Check sheet for the modelled part. Datum: model origin and axes. Units: mm. A direction names the side the tool comes from. Give positions to 0.01 mm unless a question says otherwise; leave off trailing zeros. Write each loop counter-clockwise with the first axis right and the second up, starting at its lowest first coordinate (ties: lowest second). Pieces come first, ordered by that corner, then holes. Notation, with made-up numbers: (11.5, 7.25) -> (18.5, 7.25) arc R21 ccw to (18.5, 15.25) -> close; hole circle Ø3 at (-5.75, 2). An arc over 180 degrees is marked (long way). Use a Markdown table: item, result. Add a question column.
1. Cross-section at D-D (x = 31.5). Enter the section's corners in (y, z), then the cut area to 3 significant figures.
2. Gauge pin test, flat ends, axial feed: P1, Ø8, axis at x = -16, y = 2.5, coming from the -Z side; P2, Ø12, axis at x = -20, y = 2.5, coming from the +Z side; P3, Ø12.5, axis at x = 0, y = 0, coming from the +Z side; P4, Ø1.5, axis at y = 1.5, z = 10, coming from the -X side. Record the tip position at first contact, or that the pin passes through.
3. Release check for a two-part mould opening along Y. For faces 3 (the flat face through (-16.6, -9.3, 2.3)), 4 (the flat face through (1, 8, 4.762)), 5 (the flat face through (-19, 0, 4.762)) record: released by +Y, released by -Y, zero draft, split by the parting line, or undercut.
4. Cross-section at B-B (z = 3.5). Enter the section's corners in (x, y), then the cut area to 3 significant figures.
5. Set-up check for faces 1 (the cylindrical face through (-8.88, -2.8, 2.35)), 2 (the flat face through (-8.4, -5.4, 0)): record each of +Z, -Z, +X, -X, +Y, -Y from which the full face is reachable in a straight line by a thin tool's end or side.
6. Cross-section at A-A (x = 0). Enter the section's corners in (y, z).
7. Cross-section at C-C (y = 0). Count the separate pieces of the cut face and the enclosed holes in it, then the cut area to 3 significant figures.
8. Scan lines: probe 1 along X at (y, z) = (0.75, 2); probe 2 along Z at (x, y) = (-19, 1); probe 3 along X at (y, z) = (1, 10.5). Record each from-to range of solid material in increasing order. Write a range as [from, to].
from build123d import *

# Parameters (mm, degrees)
SKETCH1_R           = 6.604
SKETCH1_R_2         = 3.429
SKETCH1_R_3         = 12.4841
SKETCH1_R_4         = 9.3091
BOSS_EXTRUDE1_DEPTH = 4.7625
SKETCH3_R           = 12.4841
SKETCH2_R           = 9.3091
SKETCH5_R           = 7.7216
CUT_EXTRUDE1_DEPTH  = 40.575251945


with BuildPart() as part:
    # Sketch1 → Boss-Extrude1 (new body)
    # profile 1 of 5: a face of its own
    with BuildSketch(Plane.XY):
        with Locations((-28.894599, 0)):
            Circle(SKETCH1_R)
        with Locations(Location((-28.894599, 0, 0), (0, 0, 180))):
            Circle(SKETCH1_R_2, mode=Mode.SUBTRACT)
    # profile 2 of 5: a face of its own
    with BuildSketch(Plane.XY):
        with BuildLine():
            Line((-2.540535565, 12.222865124), (-30.238524223, 6.465808611))
            ThreePointArc((-30.238524223, 6.465808611), (-24.727013738, 5.1228946), (-22.290599, 0))
            ThreePointArc((-22.290599, 0), (-24.727013738, -5.1228946), (-30.238524223, -6.465808611))
            Line((-30.238524223, -6.465808611), (-2.540535565, -12.222865124))
            ThreePointArc((-2.540535565, -12.222865124), (-12.4841, 0), (-2.540535565, 12.222865124))
        make_face()
    # profile 3 of 5: a face of its own
    with BuildSketch(Plane.XY):
        Circle(SKETCH1_R_3)
        with Locations(Location((0, 0, 0), (0, 0, 180))):
            Circle(SKETCH1_R_4, mode=Mode.SUBTRACT)
    # profile 4 of 5: a face of its own
    with BuildSketch(Plane.XY):
        with BuildLine():
            Line((30.238524223, 6.465808611), (2.540535565, 12.222865124))
            ThreePointArc((2.540535565, 12.222865124), (9.684241139, 7.878339062), (12.4841, 0))
            ThreePointArc((12.4841, 0), (9.684241139, -7.878339062), (2.540535565, -12.222865124))
            Line((2.540535565, -12.222865124), (30.238524223, -6.465808611))
            ThreePointArc((30.238524223, -6.465808611), (22.290599, 0), (30.238524223, 6.465808611))
        make_face()
    # profile 5 of 5: a face of its own
    with BuildSketch(Plane.XY):
        with Locations((28.894599, 0)):
            Circle(SKETCH1_R)
        with Locations(Location((28.894599, 0, 0), (0, 0, 180))):
            Circle(SKETCH1_R_2, mode=Mode.SUBTRACT)
    extrude(amount=BOSS_EXTRUDE1_DEPTH)

    # Sketch3 → Loft3 section 0
    with BuildSketch(Plane.XY.offset(4.7625)):
        Circle(SKETCH3_R)
    # Sketch2 → Loft3 section 1
    with BuildSketch(Plane.XY.offset(12.2555)):
        Circle(SKETCH2_R)
    loft()

    # Sketch5 → Cut-Extrude1 (cut, through all)
    with BuildSketch(Plane.XY.offset(12.2555)):
        Circle(SKETCH5_R)
    extrude(amount=-CUT_EXTRUDE1_DEPTH, mode=Mode.SUBTRACT)


solid = part.part
Worked answers:
| question | item | result |
|---|---|---|
| 1 | outline | (-6.07, 0) -> (-2.23, 0) -> (-2.23, 4.76) -> (-6.07, 4.76) -> close; (2.23, 0) -> (6.07, 0) -> (6.07, 4.76) -> (2.23, 4.76) -> close |
| 1 | area | 36.6 mm² |
| 2 | P1 | stops at z = 0 |
| 2 | P2 | stops at z = 4.76 |
| 2 | P3 | passes through |
| 2 | P4 | stops at x = -10.49 |
| 3 | face 3 | released by -Y |
| 3 | face 4 | undercut |
| 3 | face 5 | zero draft |
| 4 | outline | (-30.24, -6.47) -> (-2.54, -12.22) arc R12.48 ccw to (2.54, -12.22) -> (30.24, -6.47) arc R6.6 ccw to (30.24, 6.47) -> (2.54, 12.22) arc R12.48 ccw to (-2.54, 12.22) -> (-30.24, 6.47) arc R6.6 ccw to start; hole circle Ø6.86 at (-28.89, 0); hole circle Ø18.62 at (0, 0); hole circle Ø6.86 at (28.89, 0) |
| 4 | area | 917 mm² |
| 5 | face 1 | -Z |
| 5 | face 2 | -Z, +X, -X, +Y, -Y |
| 6 | outline | (-12.48, 0) -> (-9.31, 0) -> (-9.31, 4.76) -> (-7.72, 4.76) -> (-7.72, 12.26) -> (-9.31, 12.26) -> (-12.48, 4.76) -> close; (7.72, 4.76) -> (9.31, 4.76) -> (9.31, 0) -> (12.48, 0) -> (12.48, 4.76) -> (9.31, 12.26) -> (7.72, 12.26) -> close |
| 7 | separate pieces | 4 |
| 7 | enclosed holes | 0 |
| 7 | area | 232 mm² |
| 8 | probe 1 | x = [-35.46, -32.24], [-25.55, -9.28], [9.28, 25.55], [32.24, 35.46] |
| 8 | probe 2 | z = [0, 4.76] |
| 8 | probe 3 | x = [-10, -7.66], [7.66, 10] |
